from build123d import *

# Parameters (mm, degrees)
F0_R     = 35
F1_DEPTH = 150
F2_R     = 15
F3_DEPTH = 25
F4_R     = 5
F5_R     = 15
F6_DEPTH = 20
F7_SIZE  = 9.99999
F8_T     = -2.5


# Not quite as in the source:
# - a fillet or chamfer is up to 0.001 mm smaller than in the source, because OpenCascade refuses the exact size


with BuildPart() as f1:
    # F0 (on Top) → F1 (new body)
    with BuildSketch(Plane.XY):
        Circle(F0_R)
    extrude(amount=F1_DEPTH)

    # F2 (on face) → F3 (join)
    with BuildSketch(Plane.XY.offset(150)):
        Circle(F2_R)
    extrude(amount=F3_DEPTH)

    # F4
    f4_edges = [f1.edges().sort_by_distance(p)[0] for p in [
        (-35, 0, 0),
    ]]
    fillet(f4_edges, radius=F4_R)

    # F5 (on face) → F6 (cut)
    with BuildSketch(Plane(origin=(0, 0, 0), x_dir=(1, 0, 0), z_dir=(0, 0, -1))):
        Circle(F5_R)
    extrude(amount=-F6_DEPTH, mode=Mode.SUBTRACT)

    # F7 (size 10 in the source; OpenCascade refuses exactly that, so slightly less here)
    f7_edges = [f1.edges().sort_by_distance(p)[0] for p in [
        (-35, 0, 150),
        (-15, 0, 150),
    ]]
    chamfer(f7_edges, length=F7_SIZE)

    # F8
    f8_openings = [f1.faces().sort_by_distance(p)[0] for p in [
        (0, 0, 175),
    ]]
    offset(amount=F8_T, openings=f8_openings, kind=Kind.INTERSECTION)


solid = f1.part
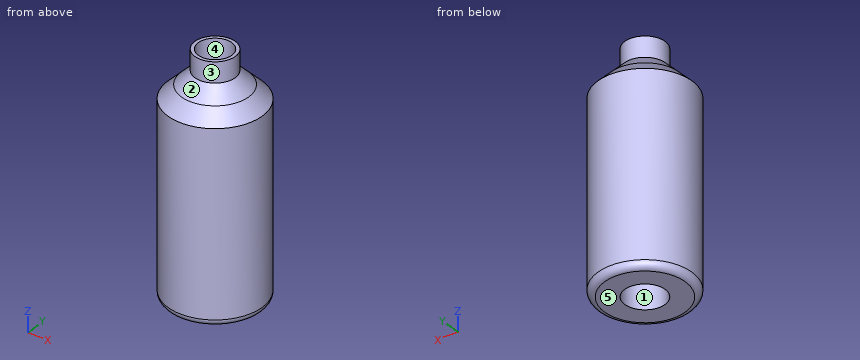
The listing builds one solid part. Answer for the finished solid, in the listing's coordinates (mm). Face numbers are marked on the shaded views. A direction names the side the tool comes from. Round coordinates to 2 decimals unless told otherwise and drop trailing zeros. Write each loop counter-clockwise with the first axis right and the second up, starting at its lowest first coordinate (ties: lowest second). Pieces come first, ordered by that corner, then holes. Notation, with made-up numbers: M 23.25,-2 L 35.25,-2 A18 ccw 35.25,4 Z; hole C -30,-8.5 d1. An arc over 180 degrees is marked long. Write each question's results on one line, items separated by ' | '. Start each with the question number.
(1) The part is cut by section A-A, the plane z = 45.5. Write down the section's boundary in (x, y), and give its area (3 significant figures).
(2) Determine the mould class of the marked faces 3, 4 and 5 for opening direction X: +X half, -X half, draft (parallel to the pull), parting line (faces both ways), or undercut.
(3) For the marked faces 1 and 2, determine the directions among +Z, -Z, +X, -X, +Y, -Y from which every point of the face is accessible in a straight line to the end or side of a thin tool.
(4) Each of these flat-tipped pins is pushed along its axis until it touches: P1, Ø3, axis at y = 26, z = 136.5, coming from the +X side (3 decimals); P2, Ø8, axis at y = -12.5, z = 52, coming from the +X side; P3, Ø5, axis at y = 20.5, z = 97, coming from the -X side. Where does it stop, or does it pass through?
(5) Find the intervals of material crossed by line 1 (X direction, y = 1.5, z = 66); line 2 (Y direction, x = 10.5, z = 14.5); line 3 (Y direction, x = 0, z = 32), in increasing order.
Worked answers:
1) outline: C 0,0 d70; hole C 0,0 d65 | area: 530 mm²
2) face 3: parting line | face 4: undercut | face 5: draft
3) face 1: -Z | face 2: +Z
4) P1: stops at x = 24.995 | P2: stops at x = 33.95 | P3: stops at x = -30.02
5) line 1: x = -34.97 to -32.47, 32.47 to 34.97 | line 2: y = -33.39 to -30.76, -14 to -10.71, 10.71 to 14, 30.76 to 33.39 | line 3: y = -35 to -32.5, 32.5 to 35
